Job drawing, mm, ordinate dimensions from the low corner. One solid piece. A direction names the side the tool comes from. Round coordinates to 2 decimals unless told otherwise and drop trailing zeros. Loops run counter-clockwise (first coordinate to the right, second up) from the corner with the lowest first, then second, coordinate; pieces in that order, holes last. Notation, with made-up numbers: M 65,63 L 93,63 A14 cw 93,68 Z; hole C 89.5,89 d8. An arc over 180 degrees is marked long. Use a Markdown table: item, result. Add a question column.
(1) Flat gauge pins, fed straight in: P1, Ø2.5, axis at x = 11, y = 1, coming from the -Z side; P2, Ø1, axis at x = 9, y = 3, coming from the +Z side; P3, Ø0.9, axis at y = 1, z = 6, coming from the -X side. Where does each tip first touch, or does it go through?
(2) Band-saw the part on D-D, the plane y = 3.65. Write the cut outline in (x, z), and give its area (3 significant figures).
(3) Wall check: L1, parallel to Z at x = 20.25, y = 2.5; L2, parallel to Z at x = 10, y = 2.85; L3, parallel to X at y = 1.25, z = 4.5. Give the ranges that are in metal, low to high.
(4) Two-plate mould, pull along Y, no slides. Class the marked faces 5, 6 and 7: released by +Y, released by -Y, zero draft, split by the parting line, or undercut.
(5) Band-saw the part on C-C, the plane z = 4.5. Write the cut outline in (x, y).
(6) Which spindle directions (+Z, -Z, +X, -X, +Y, -Y) get a long thin tool onto all of the face, cutting with end or side? Do the marked faces 1, 2, 3 and 4. Say none if no direction does.
(7) Band-saw the part on B-B, the plane x = 21. Write the cut outline in (y, z).
(8) Band-saw the part on A-A, the plane y = 0.6. Write the cut outline in (x, z).
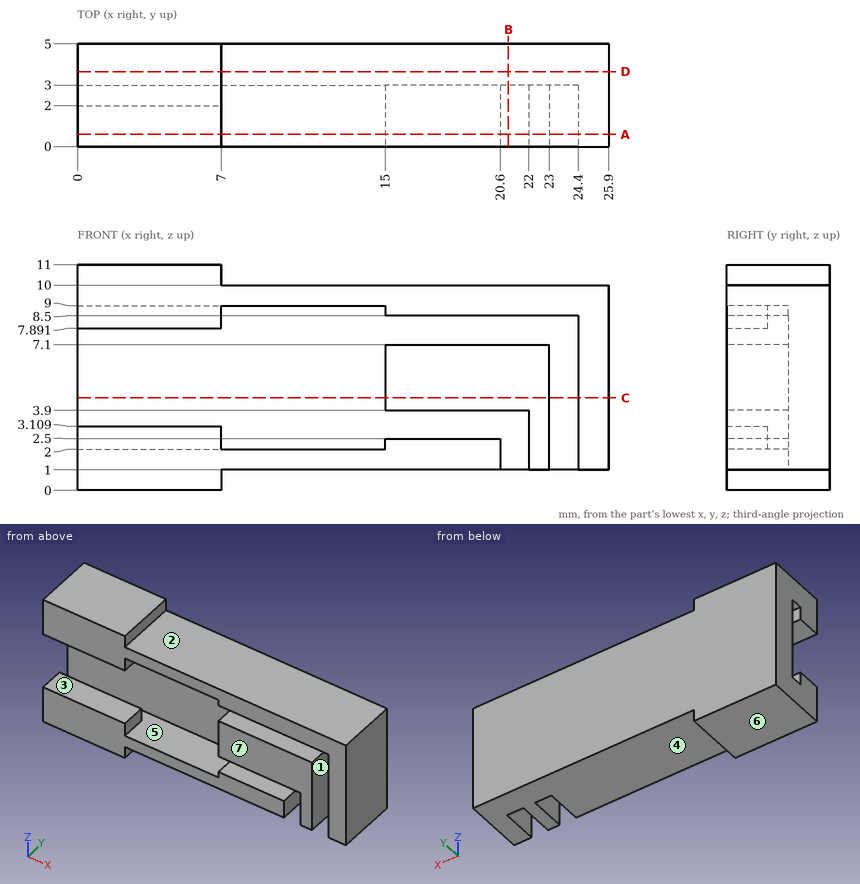
Return value:
| question | item | result |
|---|---|---|
| 1 | P1 | z = 1 |
| 1 | P2 | z = 10 |
| 1 | P3 | x = 15 |
| 2 | outline | M 0,0 L 7,0 L 7,1 L 25.9,1 L 25.9,10 L 7,10 L 7,11 L 0,11 Z |
| 2 | area | 247 mm^2 |
| 3 | L1 | 1 to 2.5, 3.9 to 7.1, 8.5 to 10 |
| 3 | L2 | 1 to 2, 9 to 10 |
| 3 | L3 | 15 to 23, 24.4 to 25.9 |
| 4 | face 5 | undercut |
| 4 | face 6 | zero draft |
| 4 | face 7 | released by -Y |
| 5 | outline | M 0,3 L 15,3 L 15,0 L 23,0 L 23,3 L 24.4,3 L 24.4,0 L 25.9,0 L 25.9,5 L 0,5 Z |
| 6 | face 1 | -Z, -Y |
| 6 | face 2 | +Z, +X, +Y, -Y |
| 6 | face 3 | -X, -Y |
| 6 | face 4 | -Z, +X, +Y, -Y |
| 7 | outline | M 0,3.9 L 3,3.9 L 3,1 L 5,1 L 5,10 L 0,10 L 0,8.5 L 3,8.5 L 3,7.1 L 0,7.1 Z |
| 8 | outline | M 0,0 L 7,0 L 7,1 L 20.6,1 L 20.6,2.5 L 15,2.5 L 15,2 L 7,2 L 7,3.11 L 0,3.11 Z; M 0,7.89 L 7,7.89 L 7,9 L 15,9 L 15,8.5 L 24.4,8.5 L 24.4,1 L 25.9,1 L 25.9,10 L 7,10 L 7,11 L 0,11 Z; M 15,3.9 L 22,3.9 L 22,1 L 23,1 L 23,7.1 L 15,7.1 Z |
